```python
from build123d import *

# Parameters (mm, degrees)
F1_DEPTH = 47
F0_W     = 40
F0_H     = 1.6352946644
F2_DEPTH = 2
F3_R     = 0.75


with BuildPart() as f1:
    # F0 (on Front) → F1 (new body)
    with BuildSketch(Plane.XZ):
        Polygon((-0.6722141189, -1.4952032847), (-0.6722141189, -8.1304979491), (43.3277858811, -8.1304979491), (43.3277858811, -1.4952032847), (41.3277858811, -1.4952032847), (41.3277858811, -3.1304979491), (1.3277858811, -3.1304979491), (1.3277858811, -1.4952032847), align=None)
    extrude(amount=F1_DEPTH)

    # F0 (on Front) → F2 (join)
    with BuildSketch(Plane.XZ):
        with Locations((21.3277858811, -2.3128506169)):
            Rectangle(F0_W, F0_H)
    extrude(amount=F2_DEPTH)

    # F3
    f3_edges = [f1.edges().sort_by_distance(p)[0] for p in [
        (1.327786, -24.5, -1.495203),
        (0.327786, -47, -1.495203),
        (-0.672214, -23.5, -1.495203),
        (21.327786, 0, -1.495203),
        (43.327786, -23.5, -1.495203),
        (42.327786, -47, -1.495203),
        (41.327786, -24.5, -1.495203),
        (21.327786, -2, -1.495203),
        (21.327786, -2, -3.130498),
        (1.327786, -24.5, -3.130498),
        (21.327786, -47, -3.130498),
        (41.327786, -24.5, -3.130498),
        (-0.672214, -23.5, -8.130498),
        (43.327786, -23.5, -8.130498),
        (21.327786, 0, -8.130498),
        (21.327786, -47, -8.130498),
        (-0.672214, 0, -4.812851),
        (43.327786, 0, -4.812851),
        (-0.672214, -47, -4.812851),
        (1.327786, -47, -2.312851),
        (43.327786, -47, -4.812851),
        (41.327786, -47, -2.312851),
    ]]
    fillet(f3_edges, radius=F3_R)


solid = f1.part
```
Could you check a few things on this model? Use its own coordinates, in mm. Coordinates: 2 decimals unless noted, no trailing zeros. Loops run counter-clockwise (first coordinate to the right, second up) from the corner with the lowest first, then second, coordinate; pieces in that order, holes last. Notation, with made-up numbers: M -19.5,49.5 L -4.5,49.5 A4 cw -4.5,56.5 Z; hole C -37,4.5 d5. An arc over 180 degrees is marked long. Put each result on its own line as item: value. Start each with the question number.
(1) Suppose I cut it at A-A on y = -12. Please give me the cut outline in (x, z).
(2) Will this pin go through, and if not, where does the flat tip stop? P1, Ø3, axis at x = 22.5, y = -4.5, coming from the +Z side.
(3) Suppose I cut it at B-B on x = 32. Please give me the cut outline in (y, z).
(4) Thinking about a two-plate mould opening in X: for faces 1 (the face through (21, 0, -5)), 2 (the face through (43.328, -23, -5)), 3 (the face through (-0.672, -23, -5)), 4 (the face through (22, -24, -3.13)), which applies, pulls with the +X half, pulls with the -X half, needs draft (parallel to the pull), parting line crosses it, or undercut?
(5) I need wall thicknesses on line 1 (X direction, y = -35.5, z = -2.5); line 2 (Z direction, x = 29.5, y = -35.5); line 3 (Y direction, x = 38, z = -2.5). Which ranges of each line are inside material? Lowest first, please. Write a range as from..to.
Solutions:
1. outline: M -0.67,-7.38 A0.75 ccw 0.08,-8.13 L 42.58,-8.13 A0.75 ccw 43.33,-7.38 L 43.33,-2.25 A0.75 ccw 42.58,-1.5 L 42.08,-1.5 A0.75 ccw 41.33,-2.25 L 41.33,-2.38 A0.75 cw 40.58,-3.13 L 2.08,-3.13 A0.75 cw 1.33,-2.38 L 1.33,-2.25 A0.75 ccw 0.58,-1.5 L 0.08,-1.5 A0.75 ccw -0.67,-2.25 Z
2. P1: stops at z = -3.13
3. outline: M -47,-7.38 A0.75 ccw -46.25,-8.13 L -0.75,-8.13 A0.75 ccw 0,-7.38 L 0,-2.25 A0.75 ccw -0.75,-1.5 L -1.25,-1.5 A0.75 ccw -2,-2.25 L -2,-2.38 A0.75 cw -2.75,-3.13 L -46.25,-3.13 A0.75 ccw -47,-3.88 Z
4. face 1: needs draft
4. face 2: pulls with the +X half
4. face 3: pulls with the -X half
4. face 4: undercut
5. line 1: x = -0.67..1.34, 41.32..43.33
5. line 2: z = -8.13..-3.13
5. line 3: y = -2.01..0
